from build123d import *

# Parameters (mm, degrees)
BOSS_EXTRUDE1_DEPTH = 6
FILLET1_R           = 1
SKETCH2_R           = 16
BOSS_EXTRUDE2_DEPTH = 0.5
SKETCH3_R           = 15
BOSS_EXTRUDE3_DEPTH = 0.5
FILLET2_SIZE        = 1
SKETCH5_R           = 3.5
CUT_EXTRUDE2_DEPTH  = 10
CIRPATTERN2_COUNT   = 4


with BuildPart() as part:
    # Sketch1 → Boss-Extrude1 (new body)
    with BuildSketch(Plane(origin=(0, 0, 0), x_dir=(1, 0, 0), z_dir=(0, 1, 0))):
        with BuildLine():
            Line((-21, -22.5), (21, -22.5))
            ThreePointArc((21, -22.5), (23.828427125, -21.328427125), (25, -18.5))
            Line((25, -18.5), (25, 18.5))
            ThreePointArc((25, 18.5), (23.828427125, 21.328427125), (21, 22.5))
            Line((21, 22.5), (-21, 22.5))
            ThreePointArc((-21, 22.5), (-23.828427125, 21.328427125), (-25, 18.5))
            Line((-25, 18.5), (-25, -18.5))
            ThreePointArc((-25, -18.5), (-23.828427125, -21.328427125), (-21, -22.5))
        make_face()
    extrude(amount=BOSS_EXTRUDE1_DEPTH)

    # Fillet1
    fillet1_edges = [part.edges().sort_by_distance(p)[0] for p in [
        (23.828427125, 6, -21.328427125),
        (0, 6, -22.5),
        (-23.828427125, 6, -21.328427125),
        (-25, 6, 0),
        (-23.828427125, 6, 21.328427125),
        (0, 6, 22.5),
        (23.828427125, 6, 21.328427125),
        (25, 6, 0),
    ]]
    fillet(fillet1_edges, radius=FILLET1_R)

    # Sketch2 → Boss-Extrude2 (add)
    with BuildSketch(Plane.XZ):
        with Locations(Location((-1.5, 0, 0), (0, 0, 270))):
            Circle(SKETCH2_R)
    extrude(amount=BOSS_EXTRUDE2_DEPTH)

    # Sketch3 → Boss-Extrude3 (add)
    with BuildSketch(Plane(origin=(0, -0.5, 0), x_dir=(-1, 0, 0), z_dir=(0, -1, 0))):
        with Locations(Location((1.5, 0, 0), (0, 0, 90))):
            Circle(SKETCH3_R)
    extrude(amount=BOSS_EXTRUDE3_DEPTH)

    # Fillet2
    # the kernel refuses this chamfer: 1 mm, written as the material it adds along each edge
    with BuildSketch(Plane(origin=(-1.5, -0.5, 0), x_dir=(0, 0, -1), z_dir=(-1, 0, 0))) as fillet2_piece_1_section:
        Polygon((15 + FILLET2_SIZE, 0), (15, FILLET2_SIZE), (15, 0), align=None)
    fillet2_piece_1 = revolve(axis=Axis((-1.5, -0.5, 0), (0, -1, 0)), mode=Mode.PRIVATE)
    fillet2_piece_1 = fillet2_piece_1 & Plane(origin=(-1.5, -0.725925615, 0), x_dir=(0, 0, -1), z_dir=(0, 1, 0)) * Cylinder(16, 64, mode=Mode.PRIVATE)
    fillet2_piece_1 = split(fillet2_piece_1, bisect_by=Plane(origin=(-1.5, -1, 15.725925615), z_dir=(0, 1, 0)), keep=Keep.TOP, mode=Mode.PRIVATE)
    add(fillet2_piece_1)

    # Sketch5 → Cut-Extrude2 (cut)
    with BuildSketch(Plane(origin=(0, 0, 0), x_dir=(-1, 0, 0), z_dir=(0, -1, 0))):
        with Locations(Location((17.763455967, 16.263455967, 0), (0, 0, 90))):
            Circle(SKETCH5_R)
    cut_extrude2 = extrude(amount=-CUT_EXTRUDE2_DEPTH, mode=Mode.SUBTRACT)

    # CirPattern2: Cut-Extrude2 ×4 about axis
    cirpattern2_axis = Axis((-1.5, 0, 0), (0, 1, 0))
    for i in range(1, CIRPATTERN2_COUNT):
        add(cut_extrude2.rotate(cirpattern2_axis, i * 360 / CIRPATTERN2_COUNT), mode=Mode.SUBTRACT)


solid = part.part
Here's how the part is built. I have some questions about the finished solid (model axes, mm). A direction names the side the tool comes from. Round coordinates to 2 decimals unless told otherwise and drop trailing zeros. Write each loop counter-clockwise with the first axis right and the second up, starting at its lowest first coordinate (ties: lowest second). Pieces come first, ordered by that corner, then holes.
1. Suppose I cut it at C-C (z = 0). List the corners of the cut face in (x, y) for me, and give its area (3 significant figures).
2. Will these pins go through, and if not, where does the flat tip stop? pin 1 Ø1 at (x, z) = (-7.5, 15.5) entering from -Y; pin 2 Ø5.5 at (x, z) = (-17.76, -16.26) entering from +Y.
3. I need wall thicknesses on L1, parallel to Z at x = 15, y = 3.5; L2, parallel to Z at x = 13.5, y = 0.5; L3, parallel to X at y = 5.5, z = 15.5. Which ranges of each line are inside material? Lowest first, please.
4. For faces 1 (the flat face through (0, 6, 0)), 2 (the cylindrical face through (-17.12, -0.25, 3.47)), which set-ups out of +Z, -Z, +X, -X, +Y, -Y let a thin tool reach every point of the face, with its end or its side?
5. Suppose I cut it at D-D (x = -1.5). List the corners of the cut face in (y, z) for me, and give its area (3 significant figures).
6. If we mould it in two halves opening along Z, with no side actions, what happens to faces 3 (the flat face through (0, 2, -22.5)), 4 (the cylindrical face through (16.38, 2.96, -19.37)), 5 (the cylindrical face through (-19.38, 2.96, 19.37)), 6 (the flat face through (0, 2, 22.5))? For each: released by +Z, released by -Z, zero draft, split by the parting line, or undercut.
7. Suppose I cut it at B-B (y = 3.75). List the corners of the cut face in (x, z) for me.
8. Suppose I cut it at A-A (x = 16). List the corners of the cut face in (y, z) for me, and give its area (3 significant figures).
Answer sheet:
1. outline: (-25, 0) - (-17.5, 0) - (-17.5, -0.5) - (-17, -1) - (14, -1) - (14.5, -0.5) - (14.5, 0) - (25, 0) - (25, 5) arc R1 ccw to (24, 6) - (-24, 6) arc R1 ccw to (-25, 5) - close
1. area: 331 mm2
2. pin 1: stops at y = 0
2. pin 2: passes through
3. L1: z = -22.5 to -19.76, -12.77 to 12.77, 19.76 to 22.5
3. L2: z = -22.5 to -19.53, -13 to 13, 19.53 to 22.5
3. L3: x = -24.87 to -21.18, -14.35 to 11.35, 18.18 to 24.87
4. face 1: +Z, -Z, +X, -X, +Y
4. face 2: -Y
5. outline: (-1, -15.5) - (-0.5, -16) - (0, -16) - (0, -22.5) - (5, -22.5) arc R1 ccw to (6, -21.5) - (6, 21.5) arc R1 ccw to (5, 22.5) - (0, 22.5) - (0, 16) - (-0.5, 16) - (-1, 15.5) - close
5. area: 301 mm2
6. face 3: released by -Z
6. face 4: undercut
6. face 5: undercut
6. face 6: released by +Z
7. outline: (-25, -18.5) arc R4 ccw to (-21, -22.5) - (21, -22.5) arc R4 ccw to (25, -18.5) - (25, 18.5) arc R4 ccw to (21, 22.5) - (-21, 22.5) arc R4 ccw to (-25, 18.5) - close; hole circle Ø7 at (-17.76, -16.26); hole circle Ø7 at (-17.76, 16.26); hole circle Ø7 at (14.76, -16.26); hole circle Ø7 at (14.76, 16.26)
8. outline: (0, -22.5) - (5, -22.5) arc R1 ccw to (6, -21.5) - (6, -19.54) - (0, -19.54) - close; (0, -12.99) - (6, -12.99) - (6, 12.99) - (0, 12.99) - close; (0, 19.54) - (6, 19.54) - (6, 21.5) arc R1 ccw to (5, 22.5) - (0, 22.5) - close
8. area: 191 mm2
